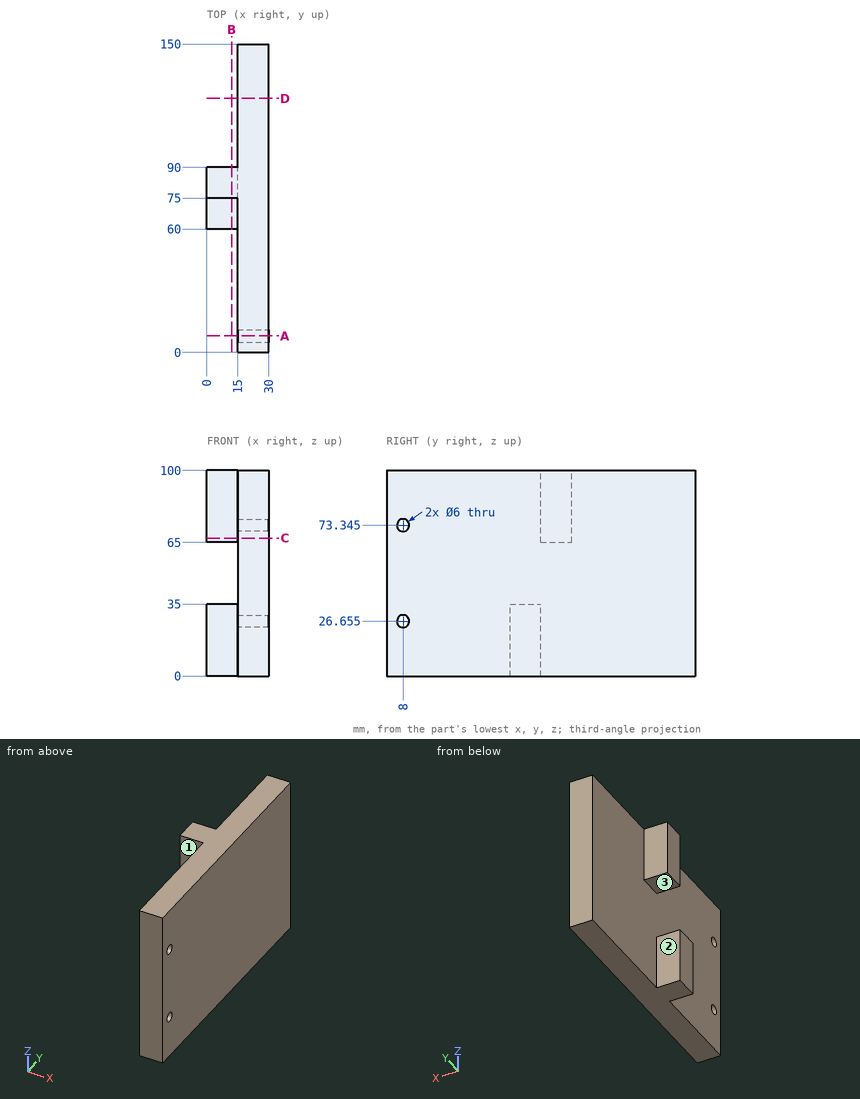
Geometry: see drawing. Coordinates: mm, zero at the bounding-box minimum. A direction names the side the tool comes from. Give positions to 0.01 mm unless a question says otherwise; leave off trailing zeros. Loops run counter-clockwise (first coordinate to the right, second up) from the corner with the lowest first, then second, coordinate; pieces in that order, holes last. Notation, with made-up numbers: (-12, 63) - (45, 63) arc R14 cw to (45, 81) - close; hole circle Ø4 at (38.25, 7). An arc over 180 degrees is marked (long way). Answer as CSV lines item,"result". Start each with the question number.
1. Reachability of the marked faces 1, 2 and 3 from +Z, -Z, +X, -X, +Y, -Y: full face, straight path, thin tool, end or side. Return the list, or none.
2. Ray query, L1, parallel to Y at x = 2, z = 81; L2, parallel to Y at x = 7.5, z = 26; L3, parallel to X at y = 110.5, z = 36.5. Return the intervals inside material, ascending.
3. Section B-B, the plane x = 12. Return loops of the section in (y, z), plus the area to 3 significant figures.
4. Section D-D, the plane y = 123.5. Return loops of the section in (x, z), plus the area to 3 significant figures.
5. Section C-C, the plane z = 67. Return loops of the section in (x, y).
6. Pin query (flat end, axial travel): P1, Ø12, axis at x = 7.5, z = 79.5, coming from the -Y side; P2, Ø1.5, axis at y = 37.5, z = 35.5, coming from the -X side; P3, Ø7.5, axis at x = 9.5, z = 9.5, coming from the +Y side. Return the tip coordinate at first contact, or that it passes through.
7. Section A-A, the plane y = 8. Return loops of the section in (x, z) (3 decimals).
Answers:
1,face 1,"+Z, -X, -Y"
1,face 2,"-Z, -X, +Y"
1,face 3,"-Z, -X, +Y, -Y"
2,L1,"y = 75 to 90"
2,L2,"y = 60 to 75"
2,L3,"x = 15 to 30"
3,outline,"(60, 0) - (75, 0) - (75, 35) - (60, 35) - close; (75, 65) - (90, 65) - (90, 100) - (75, 100) - close"
3,area,"1,050 mm2"
4,outline,"(15, 0) - (30, 0) - (30, 100) - (15, 100) - close"
4,area,"1,500 mm2"
5,outline,"(0, 75) - (15, 75) - (15, 0) - (30, 0) - (30, 150) - (15, 150) - (15, 90) - (0, 90) - close"
6,P1,"stops at y = 75"
6,P2,"stops at x = 15"
6,P3,"stops at y = 75"
7,outline,"(15, 0) - (30, 0) - (30, 23.655) - (15, 23.655) - close; (15, 29.655) - (30, 29.655) - (30, 70.345) - (15, 70.345) - close; (15, 76.345) - (30, 76.345) - (30, 100) - (15, 100) - close"
